For this review, take the finished solid that the model builds, in its own axes (mm). A direction names the side the tool comes from. Round coordinates to 2 decimals unless told otherwise and drop trailing zeros. Order: outer loops, then holes, each group sorted by start corner. A loop starts at its lowest first (then second) coordinate and runs counter-clockwise, first axis right, second up. Notation, with made-up numbers: (22.5, 55) - (73.5, 55) arc R13 cw to (73.5, 64) - close; hole circle Ø9 at (74.5, 50). An arc over 180 degrees is marked (long way). Write each question's results on one line, items separated by ' | '. Start each with the question number.
(1) For L1, parallel to Y at x = 0, z = 4.75; L2, parallel to Z at x = -4.25, y = 1.75; L3, parallel to Y at x = 3.25, z = 3.5 (3 decimals), list the stretches that pass through material, from the lowest coordinate up. Write a range as from..to.
(2) Insertion check: pin 1 Ø3 at (x, z) = (-4.5, 5.5) entering from -Y; pin 2 Ø1 at (y, z) = (5, 9) entering from -X; pin 3 Ø3 at (x, z) = (2.5, 5.5) entering from +Y. Each pin has a flat end and moves straight along its axis. Give the tip position at first contact, or say it passes through.
(3) Take a section at A-A, the plane y = 0. Give the boundary of the cut face in (x, z), plus the area to 3 significant figures.
(4) For faces 1 (the flat face through (0, 0, 8)), 2 (the flat face through (-3, -3, 0)), list the 3-axis set-ups (+Z, -Z, +X, -X, +Y, -Y) from which the entire face can be reached by the end or side of a thin tool; tool diameter is ignored.
(5) Draft analysis for pull direction Y (two halves, no side actions). For faces 3 (the flat face through (0, 0, 16)), 4 (the cylindrical face through (-3.135, -2.404, 3.944)), 5 (the cylindrical face through (-1.73, -7.81, 12.96)), state which applies: pulls with the +Y half, pulls with the -Y half, needs draft (parallel to the pull), parting line crosses it, or undercut.
(6) Take a section at C-C, the plane z = 5.75. Give the boundary of the cut face in (x, y).
(7) Take a section at D-D, the plane z = 14.25. Give the boundary of the cut face in (x, y), plus the area to 3 significant figures.
```python
from build123d import *

# Parameters (mm, degrees)
F0_R     = 4.45
F0_R_2   = 3.95
F1_DEPTH = 8
F2_R     = 4.45
F3_DEPTH = 2
F4_R     = 8
F5_DEPTH = 6


# Not quite as in the source:
# - a feature names something its author has since deleted; it is built from what else it names


with BuildPart() as f1:
    # F0 (on Top) → F1 (new body)
    with BuildSketch(Plane.XY):
        Circle(F0_R)
        Circle(F0_R_2, mode=Mode.SUBTRACT)
    extrude(amount=F1_DEPTH)

    # F2 (on face) → F3 (join)
    with BuildSketch(Plane.XY.offset(8)):
        Circle(F2_R)
    extrude(amount=F3_DEPTH)

    # F4 (on face) → F5 (join)
    with BuildSketch(Plane.XY.offset(10)):
        Circle(F4_R)
    extrude(amount=F5_DEPTH)


solid = f1.part
```
Results below:
1) L1: y = -4.45..-3.95, 3.95..4.45 | L2: z = 10..16 | L3: y = -3.04..-2.245, 2.245..3.04
2) pin 1: stops at y = -3.29 | pin 2: passes through | pin 3: stops at y = 4.34
3) outline: (-8, 10) - (-4.45, 10) - (-4.45, 0) - (-3.95, 0) - (-3.95, 8) - (3.95, 8) - (3.95, 0) - (4.45, 0) - (4.45, 10) - (8, 10) - (8, 16) - (-8, 16) - close | area: 122 mm^2
4) face 1: -Z | face 2: -Z, +X, -X, +Y, -Y
5) face 3: needs draft | face 4: undercut | face 5: parting line crosses it
6) outline: circle Ø8.9 at (0, 0); hole circle Ø7.9 at (0, 0)
7) outline: circle Ø16 at (0, 0) | area: 201 mm^2
